```python
from build123d import *

# Parameters (mm, degrees)
SKETCH1_W           = 109.475312552
SKETCH1_H           = 103.242807134
BOSS_EXTRUDE1_DEPTH = 100


# Read off the part's stored shape, not the designer's step: AdvancedHole2
with BuildPart() as part:
    # Sketch1 → Boss-Extrude1 (new body)
    with BuildSketch(Plane(origin=(0, 0, 0), x_dir=(1, 0, 0), z_dir=(0, 1, 0))):
        Rectangle(SKETCH1_W, SKETCH1_H)
    extrude(amount=BOSS_EXTRUDE1_DEPTH)

    # AdvancedHole2 outline → AdvancedHole2 (revolve, cut)
    with BuildSketch(Plane.XY):
        Polygon((9.8965, 98), (12.5, 98), (12.5, 100), (0, 100), (0, 0), (6, 0), (6, 83), (9.428250684, 83), align=None)
    revolve(axis=Axis((0, 0, 0), (0, 1, 0)), mode=Mode.SUBTRACT)


solid = part.part
```
Verification items for the finished model (mm, model axes). A direction names the side the tool comes from. Give positions to 0.01 mm unless a question says otherwise; leave off trailing zeros. Order: outer loops, then holes, each group sorted by start corner. A loop starts at its lowest first (then second) coordinate and runs counter-clockwise, first axis right, second up. Notation, with made-up numbers: M -19.5,41 L -4.5,41 A26 cw -4.5,64 Z; hole C 41.25,64 d8. An arc over 180 degrees is marked long. Answer in a Markdown table with one row per item. Add a question column.
Item 1: Tool access check on faces 5 (the flat face through (0.1, 83, 6.2)), 6 (the flat face through (-13, 100, -1)). Record the directions out of +Z, -Z, +X, -X, +Y, -Y that give a thin tool (end or side, any length) a straight path to the whole face; none if there is none.
Item 2: Section check B-B, the plane z = 0. Enter the section's corners in (x, y).
Item 3: Section check A-A, the plane x = 0. Enter the section's corners in (y, z), and give its area (3 significant figures).
Item 4: Mould release check, pull along X, two halves, no side actions. Record for faces 1 (the flat face through (-1, 98, -10)), 2 (the flat face through (-54.738, 49, 1)), 3 (the flat face through (-1, 0, -12)), 4 (the flat face through (54.738, 49, 1)): released by +X, released by -X, zero draft, split by the parting line, or undercut.
Item 5: Scan lines: probe 1 along Z at (x, y) = (0, 98.6); probe 2 along X at (y, z) = (99.05, 0); probe 3 along X at (y, z) = (36, 0). Record each from-to range of solid material in increasing order. Write a range as from..to.
Item 6: Gauge pin test, flat end, axial feed: pin 1 (20.5 mm diameter, centred on x = 1.5, z = 2.5, fed in from +Y). Record the tip position at first contact, or that the pin passes through.
Item 7: Section check C-C, the plane y = 90. Enter the section's corners in (x, z), and give its area (3 significant figures).
Filled sheet:
| question | item | result |
|---|---|---|
| 1 | face 5 | +Y |
| 1 | face 6 | +Z, -Z, +X, -X, +Y |
| 2 | outline | M -54.74,0 L -6,0 L -6,83 L -9.43,83 L -9.9,98 L -12.5,98 L -12.5,100 L -54.74,100 Z; M 6,0 L 54.74,0 L 54.74,100 L 12.5,100 L 12.5,98 L 9.9,98 L 9.43,83 L 6,83 Z |
| 3 | outline | M 0,-51.62 L 100,-51.62 L 100,-12.5 L 98,-12.5 L 98,-9.9 L 83,-9.43 L 83,-6 L 0,-6 Z; M 0,6 L 83,6 L 83,9.43 L 98,9.9 L 98,12.5 L 100,12.5 L 100,51.62 L 0,51.62 Z |
| 3 | area | 8,990 mm^2 |
| 4 | face 1 | undercut |
| 4 | face 2 | released by -X |
| 4 | face 3 | zero draft |
| 4 | face 4 | released by +X |
| 5 | probe 1 | z = -51.62..-12.5, 12.5..51.62 |
| 5 | probe 2 | x = -54.74..-12.5, 12.5..54.74 |
| 5 | probe 3 | x = -54.74..-6, 6..54.74 |
| 6 | pin 1 | stops at y = 100 |
| 7 | outline | M -54.74,-51.62 L 54.74,-51.62 L 54.74,51.62 L -54.74,51.62 Z; hole C 0,0 d19.29 |
| 7 | area | 11,000 mm^2 |
